```python
from build123d import *
from OCP.BRepFilletAPI import BRepFilletAPI_MakeChamfer

# Parameters (mm, degrees)
ESBO_O1_W                = 26
ESBO_O1_H                = 18
RESSALTO_EXTRUS_O1_DEPTH = 18
CORTE_EXTRUS_O1_DEPTH    = 33.878564446
ESBO_O3_R                = 1.25
CORTE_EXTRUS_O2_DEPTH    = 24.958297101
CHANFRO1_SIZE            = 6
CHANFRO1_SIZE2           = 3.464101615


with BuildPart() as part:
    # Esboço1 → Ressalto-extrusão1 (new body)
    with BuildSketch(Plane.XY):
        Rectangle(ESBO_O1_W, ESBO_O1_H)
    extrude(amount=RESSALTO_EXTRUS_O1_DEPTH)

    # Esboço2 → Corte-extrusão1 (cut, through all)
    with BuildSketch(Plane(origin=(13, 0, 0), x_dir=(0, 0, -1), z_dir=(1, 0, 0))):
        Polygon((-17.15, -9), (-0.85, -9), (-0.85, 1.5), (-2.187266824, 1.5), (-5.593633412, 7.4), (-12.406366588, 7.4), (-15.812733176, 1.5), (-17.15, 1.5), align=None)
    extrude(amount=-CORTE_EXTRUS_O1_DEPTH, mode=Mode.SUBTRACT)

    # Esboço3 → Corte-extrusão2 (cut, through all)
    with BuildSketch(Plane.XY.offset(18)):
        with Locations((-9, -6.1)):
            Circle(ESBO_O3_R)
        with Locations((9, -6.1)):
            Circle(ESBO_O3_R)
    extrude(amount=-CORTE_EXTRUS_O2_DEPTH, mode=Mode.SUBTRACT)

    # Chanfro1: one chamfer whose edges measure the first distance from different faces: ONE call of the kernel's chamfer builder (chamfer() names one face for all edges)
    chanfro1_edges_1 = [part.edges().sort_by_distance(p)[0] for p in [
        (0, 9, 0),
    ]]
    chanfro1_side_1 = [part.faces().sort_by_distance(p)[0] for p in [
        (0, 0.130704702, 0),
    ]]
    chanfro1_edges_2 = [part.edges().sort_by_distance(p)[0] for p in [
        (0, 9, 18),
    ]]
    chanfro1_side_2 = [part.faces().sort_by_distance(p)[0] for p in [
        (0, 0.130704702, 18),
    ]]
    chanfro1 = BRepFilletAPI_MakeChamfer(part.part.solid().wrapped)
    for e in chanfro1_edges_1:
        chanfro1.Add(CHANFRO1_SIZE, CHANFRO1_SIZE2, e.wrapped, chanfro1_side_1[0].wrapped)  # the first distance lies on this face
    for e in chanfro1_edges_2:
        chanfro1.Add(CHANFRO1_SIZE, CHANFRO1_SIZE2, e.wrapped, chanfro1_side_2[0].wrapped)  # the first distance lies on this face
    add(Compound.cast(chanfro1.Shape()), mode=Mode.REPLACE)


solid = part.part
```
Geometry: final body of the model. Coordinates: model frame, mm. A direction names the side the tool comes from. Round coordinates to 2 decimals unless told otherwise and drop trailing zeros. Order: outer loops, then holes, each group sorted by start corner. A loop starts at its lowest first (then second) coordinate and runs counter-clockwise, first axis right, second up. Notation, with made-up numbers: (0.5, 65) - (6.5, 65) arc R5 cw to (6.5, 72) - close; hole circle Ø5 at (14.5, 49). An arc over 180 degrees is marked (long way). Write item = value, one per line. Start each with the question number.
Q1. Pin query (flat end, axial travel): pin 1 (2 mm diameter, centred on x = 9, y = -6.1, fed in from +Z); pin 2 (2 mm diameter, centred on x = 0.5, z = 10, fed in from -Y); pin 3 (1.1 mm diameter, centred on x = -3, z = 16.5, fed in from -Y). Return the tip coordinate at first contact, or that it passes through.
Q2. Access query for faces 1 (the flat face through (0.182, 4.409, 3.867)), 2 (the flat face through (0, -3, 0)). Directions: +Z, -Z, +X, -X, +Y, -Y. A direction counts if a zero-diameter tool reaches every point of the face in a straight line with its end or side. Return the directions, or none.
Q3. Cut plane C-C on y = -3. Return the cut outline in (x, z).
Q4. Cut plane B-B on x = -9. Return the cut outline in (y, z).
Q5. Pull-direction query (Y, two-part tool) for faces 3 (the flat face through (0, 9, 9)), 4 (the flat face through (-13, 8, 10)), 5 (the cylindrical face through (8.079, -5.255, 17.581)); classes: +Y half, -Y half, draft (parallel to the pull), parting line (faces both ways), or undercut.
Q6. Cut plane A-A on y = -6.1. Return the cut outline in (x, z).
Q7. Cut plane D-D on x = 7. Return the cut outline in (y, z), and give its area (3 significant figures).
Q8. Ray query, line 1 (Z direction, x = -0.25, y = -0.25); line 2 (Y direction, x = 9, z = 17.75); line 3 (Y direction, x = 9, z = 17.45). Return the intervals inside material, ascending. Write a range as from..to.
Outcome:
q1.pin_1 = through
q1.pin_2 = 7.4
q1.pin_3 = 1.5
q2.face_1 = +X, -X, -Y
q2.face_2 = -Z, +X, -X, +Y, -Y
q3.outline = (-13, 0) - (13, 0) - (13, 0.85) - (-13, 0.85) - close; (-13, 17.15) - (13, 17.15) - (13, 18) - (-13, 18) - close
q4.outline = (-9, 0) - (-7.35, 0) - (-7.35, 0.85) - (-9, 0.85) - close; (-9, 17.15) - (-7.35, 17.15) - (-7.35, 18) - (-9, 18) - close; (-4.85, 0) - (3, 0) - (9, 3.46) - (9, 14.54) - (3, 18) - (-4.85, 18) - (-4.85, 17.15) - (1.5, 17.15) - (1.5, 15.81) - (7.4, 12.41) - (7.4, 5.59) - (1.5, 2.19) - (1.5, 0.85) - (-4.85, 0.85) - close
q5.face_3 = +Y half
q5.face_4 = draft
q5.face_5 = undercut
q6.outline = (-13, 0) - (-10.25, 0) - (-10.25, 0.85) - (-13, 0.85) - close; (-13, 17.15) - (-10.25, 17.15) - (-10.25, 18) - (-13, 18) - close; (-7.75, 0) - (7.75, 0) - (7.75, 0.85) - (-7.75, 0.85) - close; (-7.75, 17.15) - (7.75, 17.15) - (7.75, 18) - (-7.75, 18) - close; (10.25, 0) - (13, 0) - (13, 0.85) - (10.25, 0.85) - close; (10.25, 17.15) - (13, 17.15) - (13, 18) - (10.25, 18) - close
q7.outline = (-9, 0) - (3, 0) - (9, 3.46) - (9, 14.54) - (3, 18) - (-9, 18) - (-9, 17.15) - (1.5, 17.15) - (1.5, 15.81) - (7.4, 12.41) - (7.4, 5.59) - (1.5, 2.19) - (1.5, 0.85) - (-9, 0.85) - close
q7.area = 71.8 mm^2
q8.line_1 = 0..0.85, 17.15..18
q8.line_2 = -9..-7.35, -4.85..3.43
q8.line_3 = -9..-7.35, -4.85..3.95
